from build123d import *
from build123d.topology import SkipClean

# Parameters (mm, degrees)
SKETCH1_W               = 15
SKETCH1_H               = 35
BOSS_EXTRUDE1_DEPTH     = 2.5
CUT_EXTRUDE2_DEPTH      = 20.20286437
CUT_EXTRUDE2_DEPTH_BACK = 20.20286437
SKETCH3_W               = 4.75
SKETCH3_H               = 35
CUT_EXTRUDE3_DEPTH      = 20.20286437
FILLET1_R               = 10
CUT_EXTRUDE5_DEPTH      = 20.20286437
SKETCH7_R               = 1.6
CUT_EXTRUDE6_DEPTH      = 19.798797059
BOSS_EXTRUDE2_DEPTH     = 5.499997748
CUT_EXTRUDE7_START      = -0.95
CUT_EXTRUDE7_DEPTH      = 3.6
SKETCH11_R              = 5.25
CUT_EXTRUDE8_DEPTH      = 24.068697681
CHAMFER1_SIZE           = 1
FILLET2_R               = 1


with BuildPart() as part:
    # Sketch1 → Boss-Extrude1 (new body)
    with BuildSketch(Plane(origin=(0, 0, 0), x_dir=(1, 0, 0), z_dir=(0, 1, 0))):
        Rectangle(SKETCH1_W, SKETCH1_H)
    extrude(amount=BOSS_EXTRUDE1_DEPTH)

    # Sketch3 → Cut-Extrude2 (cut, two sides: drawn at the far end of the back side and taken through both)
    with BuildSketch(Plane.XZ.offset(-CUT_EXTRUDE2_DEPTH_BACK)):
        with Locations((5.125, 0)):
            Rectangle(SKETCH3_W, SKETCH3_H)
    extrude(amount=CUT_EXTRUDE2_DEPTH + CUT_EXTRUDE2_DEPTH_BACK, mode=Mode.SUBTRACT)

    # Sketch5 → Cut-Extrude3 (cut, through all)
    with BuildSketch(Plane(origin=(0, 2.5, 0), x_dir=(1, 0, 0), z_dir=(0, 1, 0))):
        with BuildLine():
            Line((-5.749997748, -12), (-10.249997748, -12))
            ThreePointArc((-10.249997748, -12), (-12.371318091, -11.121320344), (-13.249997748, -9))
            Line((-13.249997748, -9), (-13.249997748, 9))
            ThreePointArc((-13.249997748, 9), (-12.371318091, 11.121320344), (-10.249997748, 12))
            Line((-10.249997748, 12), (-5.749997748, 12))
            ThreePointArc((-5.749997748, 12), (-3.628677404, 11.121320344), (-2.749997748, 9))
            Line((-2.749997748, 9), (-2.749997748, -9))
            ThreePointArc((-2.749997748, -9), (-3.628677404, -11.121320344), (-5.749997748, -12))
        make_face()
    extrude(amount=-CUT_EXTRUDE3_DEPTH, mode=Mode.SUBTRACT)

    # Fillet1
    # the kernel refuses this fillet: 10 mm, written as the material it takes off along each edge
    with BuildSketch(Plane(origin=(-7.5, -22.325713874, 17.5), x_dir=(1, 0, 0), z_dir=(0, 1, 0))) as fillet1_piece_1:
        with BuildLine():
            CenterArc((8.93028555, 10), FILLET1_R, 206.74368395, 63.25631605)
            Line((0, 5.5), (-0.178605711, 5.41))
            ThreePointArc((-0.178605711, 5.41), (-0.2, 2.75), (-0.2, 0))
            Line((-0.2, 0), (0, -0.2))
            Line((0, -0.2), (8.93028555, -0.2))
            Line((8.93028555, -0.2), (8.93028555, 0))
        make_face()
    extrude(amount=47.151427749, mode=Mode.SUBTRACT)
    with BuildSketch(Plane(origin=(-7.5, -22.325713874, -17.5), x_dir=(1, 0, 0), z_dir=(0, 1, 0))) as fillet1_piece_2:
        with BuildLine():
            CenterArc((8.93028555, -10), FILLET1_R, 90, 63.25631605)
            Line((0, -5.5), (-0.178605711, -5.41))
            ThreePointArc((-0.178605711, -5.41), (-0.2, -2.75), (-0.2, 0))
            Line((-0.2, 0), (0, 0.2))
            Line((0, 0.2), (8.93028555, 0.2))
            Line((8.93028555, 0.2), (8.93028555, 0))
        make_face()
    extrude(amount=47.151427749, mode=Mode.SUBTRACT)

    # Sketch6 → Cut-Extrude5 (cut, through all)
    with BuildSketch(Plane(origin=(0, 2.5, 0), x_dir=(1, 0, 0), z_dir=(0, 1, 0))):
        with BuildLine():
            Line((1.43028555, 17.2), (2.75, 17.2))
            Line((2.75, 17.2), (2.75, 17.5))
            Line((2.75, 17.5), (1.43028555, 17.5))
            ThreePointArc((1.43028555, 17.5), (-3.813758691, 16.014693183), (-7.5, 12))
            Line((-7.5, 12), (-7.162734874, 12))
            ThreePointArc((-7.162734874, 12), (-3.591666262, 15.798795093), (1.43028555, 17.2))
        make_face()
        with BuildLine():
            Line((2.75, -17.5), (2.75, -17.2))
            Line((2.75, -17.2), (1.43028555, -17.2))
            ThreePointArc((1.43028555, -17.2), (-3.591666262, -15.798795093), (-7.162734874, -12))
            Line((-7.162734874, -12), (-7.5, -12))
            ThreePointArc((-7.5, -12), (-3.813758691, -16.014693183), (1.43028555, -17.5))
            Line((1.43028555, -17.5), (2.75, -17.5))
        make_face()
    extrude(amount=-CUT_EXTRUDE5_DEPTH, mode=Mode.SUBTRACT)

    # Sketch7 → Cut-Extrude6 (cut, through all)
    with BuildSketch(Plane(origin=(0, 2.5, 0), x_dir=(1, 0, 0), z_dir=(0, 1, 0))):
        with Locations(Location((-0.5, 12, 0), (0, 0, 270))):
            Circle(SKETCH7_R)
        with Locations(Location((-0.5, -12, 0), (0, 0, 270))):
            Circle(SKETCH7_R)
    extrude(amount=-CUT_EXTRUDE6_DEPTH, mode=Mode.SUBTRACT)

    # Sketch9 → Boss-Extrude2 (add)
    with BuildSketch(Plane(origin=(2.75, 0, 0), x_dir=(0, 0, -1), z_dir=(1, 0, 0))):
        with BuildLine():
            Line((-8, 2.5), (-5.015974482, 2.5))
            ThreePointArc((-5.015974482, 2.5), (-0.783783762, 9.241163936), (5.25, 4.05))
            ThreePointArc((5.25, 4.05), (5.191163936, 3.266216238), (5.015974482, 2.5))
            Line((5.015974482, 2.5), (8, 2.5))
            Line((8, 2.5), (8, 4.25))
            ThreePointArc((8, 4.25), (5.803300859, 9.553300859), (0.5, 11.75))
            Line((0.5, 11.75), (-0.5, 11.75))
            ThreePointArc((-0.5, 11.75), (-5.803300859, 9.553300859), (-8, 4.25))
            Line((-8, 4.25), (-8, 2.5))
        make_face()
    extrude(amount=-BOSS_EXTRUDE2_DEPTH)

    # Sketch10 → Cut-Extrude7 (cut)
    with BuildSketch(Plane(origin=(2.75, 0, 0), x_dir=(0, 0, -1), z_dir=(1, 0, 0)).offset(CUT_EXTRUDE7_START)):
        with BuildLine():
            ThreePointArc((6.1, 4.05), (0, 10.15), (-6.1, 4.05))
            ThreePointArc((-6.1, 4.05), (-5.70242473, 1.883816212), (-4.561523868, 0))
            Line((-4.561523868, 0), (-3.340658618, 0))
            ThreePointArc((-3.340658618, 0), (-4.361287561, 1.127386305), (-5.015974482, 2.5))
            ThreePointArc((-5.015974482, 2.5), (-0.783783762, 9.241163936), (5.25, 4.05))
            ThreePointArc((5.25, 4.05), (5.191163936, 3.266216238), (5.015974482, 2.5))
            ThreePointArc((5.015974482, 2.5), (4.361287561, 1.127386305), (3.340658618, 0))
            Line((3.340658618, 0), (4.561523868, 0))
            ThreePointArc((4.561523868, 0), (5.70242473, 1.883816212), (6.1, 4.05))
        make_face()
        with BuildLine():
            ThreePointArc((-4.561523868, 0), (-5.70242473, 1.883816212), (-6.1, 4.05))
            Line((-6.1, 4.05), (-6.1, 0))
            Line((-6.1, 0), (-4.561523868, 0))
        make_face()
        with BuildLine():
            Line((6.1, 0), (6.1, 4.05))
            ThreePointArc((6.1, 4.05), (5.70242473, 1.883816212), (4.561523868, 0))
            Line((4.561523868, 0), (6.1, 0))
        make_face()
    extrude(amount=-CUT_EXTRUDE7_DEPTH, mode=Mode.SUBTRACT)

    # Sketch11 → Cut-Extrude8 (cut, through all)
    with SkipClean():  # the faces are left unmerged after this step: merging them gives an invalid solid
        with BuildSketch(Plane(origin=(2.75, 0, 0), x_dir=(0, 0, -1), z_dir=(1, 0, 0))):
            with Locations((0, 4.05)):
                Circle(SKETCH11_R)
        extrude(amount=-CUT_EXTRUDE8_DEPTH, mode=Mode.SUBTRACT)

    # Chamfer1
    chamfer1_edges = [part.edges().sort_by_distance(p)[0] for p in [
        (1.126e-06, 2.5, 8),
        (1.126e-06, 2.5, -8),
    ]]
    chamfer(chamfer1_edges, length=CHAMFER1_SIZE)

    # Fillet2
    fillet2_edges = [part.edges().sort_by_distance(p)[0] for p in [
        (1.126e-06, 3.5, 8),
        (1.126e-06, 2.5, 9),
        (1.126e-06, 2.5, -9),
        (1.126e-06, 3.5, -8),
    ]]
    fillet(fillet2_edges, radius=FILLET2_R)


solid = part.part
Part model, mm, in its own coordinate system. A direction names the side the tool comes from. Round coordinates to 2 decimals unless told otherwise and drop trailing zeros. Write each loop counter-clockwise with the first axis right and the second up, starting at its lowest first coordinate (ties: lowest second). Pieces come first, ordered by that corner, then holes. Notation, with made-up numbers: (-29.5, 22.5) - (-5.5, 22.5) arc R30 cw to (-5.5, 50.5) - close; hole circle Ø6 at (-13.5, 30.5). An arc over 180 degrees is marked (long way). Use CSV: the item, a comma, the result in double quotes.
Item 1: Tool access for faces 4 (the flat face through (2.75, 2, -5)), 5 (the flat face through (-1, 2.5, -14)), 6 (the flat face through (1.8, 9.6, 0)), 7 (the flat face through (-6, 1, -12)): list every direction of +Z, -Z, +X, -X, +Y, -Y with a clear straight run to the whole face (end or side of a thin tool).
Results list:
face 4,"+Z, -Z, +X, +Y, -Y"
face 5,"-Z, +X, -X, +Y"
face 6,"-Y"
face 7,"-X, +Y, -Y"
Item 2: Flat gauge pins, fed straight in: P1, Ø0.7, axis at x = -6.5, y = 2, coming from the +Z side; P2, Ø3.5, axis at y = 5, z = -3.5, coming from the -X side; P3, Ø2.5, axis at x = -1, z = 13.5, coming from the +Y side; P4, Ø4, axis at x = 0, y = 1.5, coming from the +Z side. Where does each tip first touch, or does it go through?
Results list:
P1,"stops at z = 13.55"
P2,"stops at x = -2.75"
P3,"stops at y = 2.5"
P4,"stops at z = 17.2"
Item 3: Slice it at C-C, the plane z = 0. Write the cut outline in (x, y), then the cut area to 3 significant figures.
Results list:
outline,"(-2.75, 9.3) - (-1.8, 9.3) - (-1.8, 10.15) - (1.8, 10.15) - (1.8, 9.3) - (2.75, 9.3) - (2.75, 11.75) - (-2.75, 11.75) - close"
area,"10.4 mm²"
Item 4: Slice it at A-A, the plane y = 7.5. Write the cut outline in (x, z).
Results list:
outline,"(-2.75, -7.26) - (2.75, -7.26) - (2.75, -3.96) - (1.8, -3.96) - (1.8, -5.03) - (-1.8, -5.03) - (-1.8, -3.96) - (-2.75, -3.96) - close; (-2.75, 3.96) - (-1.8, 3.96) - (-1.8, 5.03) - (1.8, 5.03) - (1.8, 3.96) - (2.75, 3.96) - (2.75, 7.26) - (-2.75, 7.26) - close"
Item 5: Pull direction X, two halves, no side cores. Call faces 1 (the cylindrical face through (-0.43, 1.27, 10.4)), 2 (the cylindrical face through (0.039, 9.495, -5.861)), 3 (the cylindrical face through (-3.61, 1.31, 11.1)): pulls with the +X half, pulls with the -X half, needs draft (parallel to the pull), parting line crosses it, or undercut.
Results list:
face 1,"undercut"
face 2,"needs draft"
face 3,"pulls with the -X half"
Item 6: Slice it at D-D, the plane y = 9.75. Write the cut outline in (x, z), then the cut area to 3 significant figures.
Results list:
outline,"(-2.75, -5.6) - (2.75, -5.6) - (2.75, 5.6) - (-2.75, 5.6) - close; hole (-1.8, -2.17) - (1.8, -2.17) - (1.8, 2.17) - (-1.8, 2.17) - close"
area,"45.9 mm²"
Item 7: Slice it at B-B, the plane x = -0.5. Write the cut outline in (y, z), then the cut area to 3 significant figures.
Results list:
outline,"(0, -17.01) - (2.5, -17.01) - (2.5, -13.6) - (0, -13.6) - close; (0, -10.4) - (2.5, -10.4) - (2.5, -9.41) arc R1 cw to (2.79, -8.71) - (3.21, -8.29) arc R1 cw to (3.91, -8) - (4.25, -8) arc R7.5 ccw to (11.75, -0.5) - (11.75, 0.5) arc R7.5 ccw to (4.25, 8) - (3.91, 8) arc R1 cw to (3.21, 8.29) - (2.79, 8.71) arc R1 cw to (2.5, 9.41) - (2.5, 10.4) - (0, 10.4) - (0, 6.1) - (4.05, 6.1) arc R6.1 cw to (4.05, -6.1) - (0, -6.1) - close; (0, 13.6) - (2.5, 13.6) - (2.5, 17.01) - (0, 17.01) - close"
area,"86.1 mm²"
Item 8: Wall check: L1, parallel to Z at x = -2.35, y = 4.05; L2, parallel to Z at x = -4.25, y = 2.25; L3, parallel to Y at x = -5, z = -13. Give the ranges that are in metal, low to high.
Results list:
L1,"z = -8 to -5.25, 5.25 to 8"
L2,"z = -15.36 to -11.6, 11.6 to 15.36"
L3,"y = 0 to 2.5"
